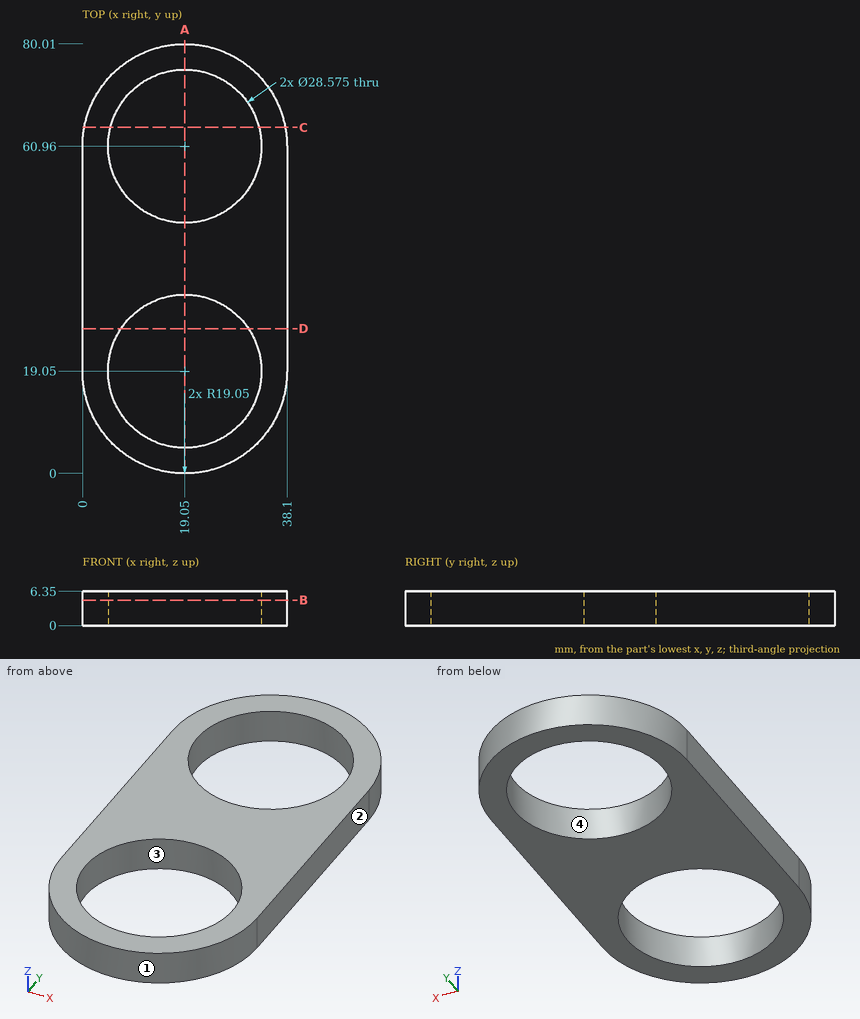
Input: dimensioned drawing with shaded views. Units: mm. Origin: part minimum x, y, z. Coordinates: 2 decimals unless noted, no trailing zeros. Loops run counter-clockwise (first coordinate to the right, second up) from the corner with the lowest first, then second, coordinate; pieces in that order, holes last.
Q1. Section D-D, the plane y = 27. Return the cut outline in (x, z), and give its area (3 significant figures).
Results are:
outline: (0, 0) - (7.18, 0) - (7.18, 6.35) - (0, 6.35) - close; (30.92, 0) - (38.1, 0) - (38.1, 6.35) - (30.92, 6.35) - close
area: 91.2 mm2
Q2. Section C-C, the plane y = 64.5. Return the cut outline in (x, z), and give its area (3 significant figures).
Results are:
outline: (0.33, 0) - (5.21, 0) - (5.21, 6.35) - (0.33, 6.35) - close; (32.89, 0) - (37.77, 0) - (37.77, 6.35) - (32.89, 6.35) - close
area: 61.9 mm2
Q3. Line query: line 1 along Y through (x, z) = (19.05, 4.25); line 2 along Y through (x, z) = (30.5, 2.5); line 3 along X through (y, z) = (19, 0.75). Output: solid intervals per line, ascending.
Results are:
line 1: y = 0 to 4.76, 33.34 to 46.67, 75.25 to 80.01
line 2: y = 3.83 to 10.5, 27.6 to 52.41, 69.51 to 76.18
line 3: x = 0 to 4.76, 33.34 to 38.1
Q4. Contact query for flat-ended pins moving along their axis: pin 1 (12 mm diameter, centred on x = 32, y = 38, fed in from -Z); pin 2 (3 mm diameter, centred on x = 23, z = 3, fed in from -Y); pin 3 (1 mm diameter, centred on y = 10.5, z = 5.5, fed in from +X). Output: stop coordinate, or through.
Results are:
pin 1: stops at z = 0
pin 2: stops at y = 0.16
pin 3: stops at x = 36.32
Q5. Section A-A, the plane x = 19.05. Return the cut outline in (y, z), and give its area (3 significant figures).
Results are:
outline: (0, 0) - (4.76, 0) - (4.76, 6.35) - (0, 6.35) - close; (33.34, 0) - (46.67, 0) - (46.67, 6.35) - (33.34, 6.35) - close; (75.25, 0) - (80.01, 0) - (80.01, 6.35) - (75.25, 6.35) - close
area: 145 mm2
Q6. Section B-B, the plane z = 4.75. Give the number of separate pieces and of enclosed holes in the cut face, and give its area (3 significant figures).
Results are:
separate pieces: 1
enclosed holes: 2
area: 1,450 mm2
Q7. Mould query, pull axis X, two halves, no side actions, for the marked faces 1, 2, 3 and 4. Classes: +X half, -X half, draft (parallel to the pull), parting line (faces both ways), or undercut.
Results are:
face 1: parting line
face 2: +X half
face 3: undercut
face 4: undercut
